Part model, mm, in its own coordinate system. Coordinates: 2 decimals unless noted, no trailing zeros. Order: outer loops, then holes, each group sorted by start corner. A loop starts at its lowest first (then second) coordinate and runs counter-clockwise, first axis right, second up. Notation, with made-up numbers: (37, 43) - (73, 43) arc R16 cw to (73, 58) - close; hole circle Ø5 at (-20, -9). An arc over 180 degrees is marked (long way). Use a Markdown table: item, result. Add a question column.
1) Two-plate mould, pull along X, no slides. Class faces 1 (the face through (188.642, 125.547, 3.131)), 2 (the face through (254, 88, 3)), 3 (the face through (125, 90, 6.35)), 4 (the face through (185.47, 89.56, 3.13)): +X half, -X half, draft (parallel to the pull), parting line (faces both ways), or undercut.
2) Saw through at A-A on y = 139.7. List the corners of the cut face in (x, z).
3) Saw through at B-B on z = 4.5. List the corners of the cut face in (x, y).
4) Saw through at C-C on y = 72. List the corners of the cut face in (x, z), then the cut area to 3 significant figures.
5) Wall check: L1, parallel to Y at x = 177.8, z = 1.5; L2, parallel to X at y = 26, z = 3.25; L3, parallel to X at y = 112, z = 5.5. Give the ranges that are in metal, low to high. Write a range as [from, to].
Autodesk Fusion 360 part; units mm, degrees
sketch "Sketch1" plane through (0, 0, 0) normal (0, 0, 1) x (1, 0, 0)
  line L0 (0, 0) -> (254, 0)
  line L1 (254, 0) -> (254, 177.8)
  line L2 (254, 177.8) -> (0, 177.8)
  line L3 (0, 177.8) -> (0, 0)
  circle A0 centre (177.8, 50.8) radius 14.2748
  circle A1 centre (205.2911, 77.9517) radius 14.2748
  circle A2 centre (177.8, 101.6) radius 14.2748
  circle A3 centre (152.4, 25.4) radius 14.2748
  circle A4 centre (190.5, 139.7) radius 14.2748
  dimension "d1" = 254
  dimension "d2" = 177.8
  dimension "d3" = 28.5496
  dimension "d4" = 177.8
  dimension "d5" = 50.8
  dimension "d6" = 28.5496
  dimension "d7" = 28.5496
  dimension "d8" = 28.5496
  dimension "d9" = 28.5496
extrude "Extrude1" add sketch "Sketch1" along normal blind 6.35
Results are:
| question | item | result |
|---|---|---|
| 1 | face 1 | undercut |
| 1 | face 2 | +X half |
| 1 | face 3 | draft |
| 1 | face 4 | undercut |
| 2 | outline | (0, 0) - (176.23, 0) - (176.23, 6.35) - (0, 6.35) - close; (204.77, 0) - (254, 0) - (254, 6.35) - (204.77, 6.35) - close |
| 3 | outline | (0, 0) - (254, 0) - (254, 177.8) - (0, 177.8) - close; hole circle Ø28.55 at (152.4, 25.4); hole circle Ø28.55 at (177.8, 50.8); hole circle Ø28.55 at (177.8, 101.6); hole circle Ø28.55 at (190.5, 139.7); hole circle Ø28.55 at (205.29, 77.95) |
| 4 | outline | (0, 0) - (192.32, 0) - (192.32, 6.35) - (0, 6.35) - close; (218.27, 0) - (254, 0) - (254, 6.35) - (218.27, 6.35) - close |
| 4 | area | 1,450 mm2 |
| 5 | L1 | [0, 36.53], [65.07, 87.33], [115.87, 133.18], [146.22, 177.8] |
| 5 | L2 | [0, 138.14], [166.66, 254] |
| 5 | L3 | [0, 168.02], [187.58, 254] |
